The listing builds one solid part. Answer for the finished solid, in the listing's coordinates (mm). A direction names the side the tool comes from. Give positions to 0.01 mm unless a question says otherwise; leave off trailing zeros. Write each loop counter-clockwise with the first axis right and the second up, starting at its lowest first coordinate (ties: lowest second). Pieces come first, ordered by that corner, then holes. Notation, with made-up numbers: (-21.75, 54.25) - (3.25, 54.25) arc R14 ccw to (3.25, 59.25) - close; hole circle Ø5 at (79.25, 63). An arc over 180 degrees is marked (long way). Return JSON: item names as keys, results as strings.
from build123d import *

# Parameters (mm, degrees)
SKETCH1_R           = 9
BOSS_EXTRUDE1_DEPTH = 7
SKETCH2_R           = 2.5
CUT_EXTRUDE4_DEPTH  = 11
CUT_EXTRUDE5_START  = -14
CUT_EXTRUDE5_DEPTH  = 14
CUT_EXTRUDE6_DEPTH  = 1


with BuildPart() as part:
    # Sketch1 → Boss-Extrude1 (new body)
    with BuildSketch(Plane(origin=(0, 0, 0), x_dir=(1, 0, 0), z_dir=(0, 1, 0))):
        with Locations(Location((0, 0, 0), (0, 0, 270))):
            Circle(SKETCH1_R)
    extrude(amount=BOSS_EXTRUDE1_DEPTH)

    # Sketch2 → Cut-Extrude4 (cut)
    with BuildSketch(Plane(origin=(0, 7, 0), x_dir=(1, 0, 0), z_dir=(0, 1, 0))):
        with Locations(Location((0, 0, 0), (0, 0, 270))):
            Circle(SKETCH2_R)
    extrude(amount=-CUT_EXTRUDE4_DEPTH, mode=Mode.SUBTRACT)

    # Sketch16 → Cut-Extrude5 (cut)
    with BuildSketch(Plane(origin=(0, 7, 0), x_dir=(1, 0, 0), z_dir=(0, 1, 0)).offset(CUT_EXTRUDE5_START)):
        with BuildLine():
            Line((2.282849902, -1.019115461), (-2.5, 0))
            Line((-2.5, 0), (-9, 0))
            ThreePointArc((-9, 0), (-1.877482723, -8.801991742), (8.216679694, -3.672352761))
            ThreePointArc((8.216679694, -3.672352761), (8.217469862, -3.670584296), (8.218259648, -3.66881566))
            Line((8.218259648, -3.66881566), (2.282849902, -1.019115461))
        make_face()
    extrude(amount=CUT_EXTRUDE5_DEPTH, mode=Mode.SUBTRACT)

    # Sketch23 → Cut-Extrude6 (cut)
    with BuildSketch(Plane(origin=(0, 7, 0), x_dir=(1, 0, 0), z_dir=(0, 1, 0))):
        with BuildLine():
            ThreePointArc((3, 0), (0, 3), (-3, 0))
            Line((-3, 0), (-2.5, 0))
            ThreePointArc((-2.5, 0), (0, 2.5), (2.5, 0))
            Line((2.5, 0), (3, 0))
        make_face()
    extrude(amount=-CUT_EXTRUDE6_DEPTH, mode=Mode.SUBTRACT)


solid = part.part
Item 1: Consider L1, parallel to Z at x = 0, y = 2; L2, parallel to X at y = 4.5, z = -3.5; L3, parallel to Z at x = 0.75, y = 4.5. Determine where each line is inside the solid, lowest interval first.
Answer below:
{"L1": "z = -9 to -2.5", "L2": "x = -8.29 to 8.29", "L3": "z = -8.97 to -2.38"}
Item 2: A cutting plane is placed at A-A on z = -2. Determine the outline of the cut face in (x, y).
Answer below:
{"outline": "(-8.77, 0) - (-1.5, 0) - (-1.5, 6) - (-2.24, 6) - (-2.24, 7) - (-8.77, 7) - close; (1.5, 0) - (8.77, 0) - (8.77, 7) - (2.24, 7) - (2.24, 6) - (1.5, 6) - close"}
Item 3: A cutting plane is placed at D-D on z = -8. Determine the outline of the cut face in (x, y).
Answer below:
{"outline": "(-4.12, 0) - (4.12, 0) - (4.12, 7) - (-4.12, 7) - close"}
Item 4: A cutting plane is placed at B-B on x = 0. Determine the outline of the cut face in (y, z), then the cut area to 3 significant figures.
Answer below:
{"outline": "(0, -9) - (7, -9) - (7, -3) - (6, -3) - (6, -2.5) - (0, -2.5) - close", "area": "45.0 mm²"}
Item 5: For faces 4 (the face through (-6, 3, 0)), 5 (the face through (0.1, 6.5, -3)), 6 (the face through (0, 7, -4)), determine the directions among +Z, -Z, +X, -X, +Y, -Y from which every point of the face is accessible in a straight line to the end or side of a thin tool.
Answer below:
{"face 4": "+Z, -X, +Y, -Y", "face 5": "+Y", "face 6": "+Z, -Z, +X, -X, +Y"}
Item 6: A cutting plane is placed at C-C on y = 3. Determine the outline of the cut face in (x, z).
Answer below:
{"outline": "(-9, 0) arc R9 ccw (long way) to (8.22, 3.67) - (2.28, 1.02) arc R2.5 cw (long way) to (-2.5, 0) - close"}
Item 7: The mould has two halves that part along Z. Classify faces 1 (the face through (0, 0, -3)), 2 (the face through (5.29, 3.45, 2.36)), 3 (the face through (-0.46, 6, -2.62)): +Z half, -Z half, draft (parallel to the pull), parting line (faces both ways), or undercut.
Answer below:
{"face 1": "draft", "face 2": "+Z half", "face 3": "undercut"}
Item 8: Flat-ended cylindrical pins translate along their axes: P1, Ø4, axis at y = 4.5, z = -7, coming from the +X side; P2, Ø1.5, axis at x = -0.5, z = -5.5, coming from the -Y side; P3, Ø1, axis at x = -6, y = 1.5, coming from the +Z side; P4, Ø1, axis at x = 3, y = 1, coming from the +Z side. Find the tip coordinate at first contact, or state that the pin passes through.
Answer below:
{"P1": "stops at x = 7.48", "P2": "stops at y = 0", "P3": "stops at z = 0", "P4": "stops at z = 1.56"}
